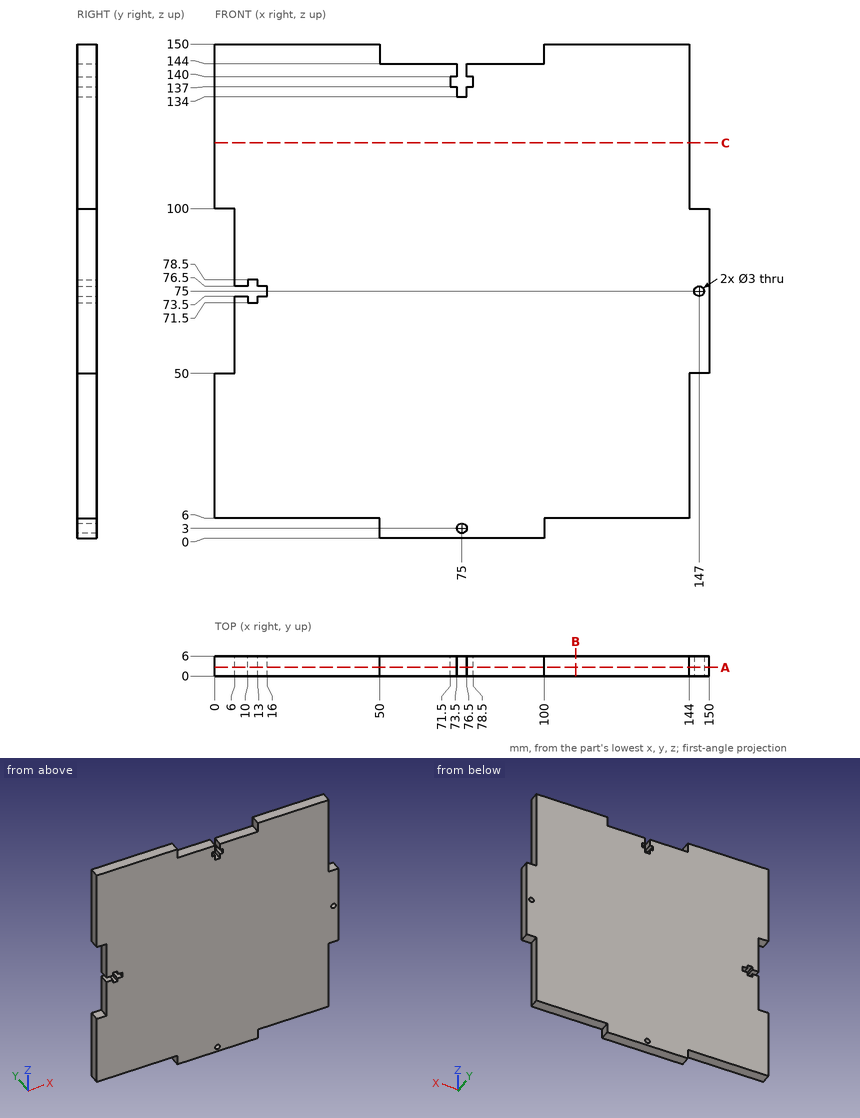
Input: dimensioned drawing with shaded views. Units: mm. Origin: part minimum x, y, z. Round coordinates to 2 decimals unless told otherwise and drop trailing zeros. Loops run counter-clockwise (first coordinate to the right, second up) from the corner with the lowest first, then second, coordinate; pieces in that order, holes last. Notation, with made-up numbers: M 29,62.5 L 33,62.5 A28 cw 33,84.5 Z; hole C 17,50.25 d5. An arc over 180 degrees is marked long. Answer in a Markdown table with one row per item. Add a question column.
1. Ray query, probe 1 along Z at (x, y) = (147, 3.15); probe 2 along X at (y, z) = (2.5, 75); probe 3 along X at (y, z) = (3.15, 14.5). Return the intervals inside material, ascending.
2. Contact query for flat-ended pins moving along their axis: pin 1 (3 mm diameter, centred on y = 4, z = 146.5, fed in from +X); pin 2 (3.5 mm diameter, centred on x = 14, y = 4.5, fed in from -Z); pin 3 (3.5 mm diameter, centred on y = 2, z = 75, fed in from -X); pin 4 (2.5 mm diameter, centred on x = 75, z = 3, fed in from +Y). Output: stop coordinate, or through.
3. Section B-B (x = 109.5). Output: boundary loops of the cut face in (y, z).
4. Section C-C (z = 120). Output: boundary loops of the cut face in (x, y).
5. Section A-A (y = 2.6). Give the number of separate pieces and of enclosed holes in the cut face, and give its area (3 significant figures).
Values follow:
| question | item | result |
|---|---|---|
| 1 | probe 1 | 50 to 73.5, 76.5 to 100 |
| 1 | probe 2 | 16 to 145.5, 148.5 to 150 |
| 1 | probe 3 | 0 to 144 |
| 2 | pin 1 | x = 144 |
| 2 | pin 2 | z = 6 |
| 2 | pin 3 | x = 6 |
| 2 | pin 4 | through |
| 3 | outline | M 0,6 L 6,6 L 6,150 L 0,150 Z |
| 4 | outline | M 0,0 L 144,0 L 144,6 L 0,6 Z |
| 5 | separate pieces | 1 |
| 5 | enclosed holes | 2 |
| 5 | area | 20,600 mm^2 |
